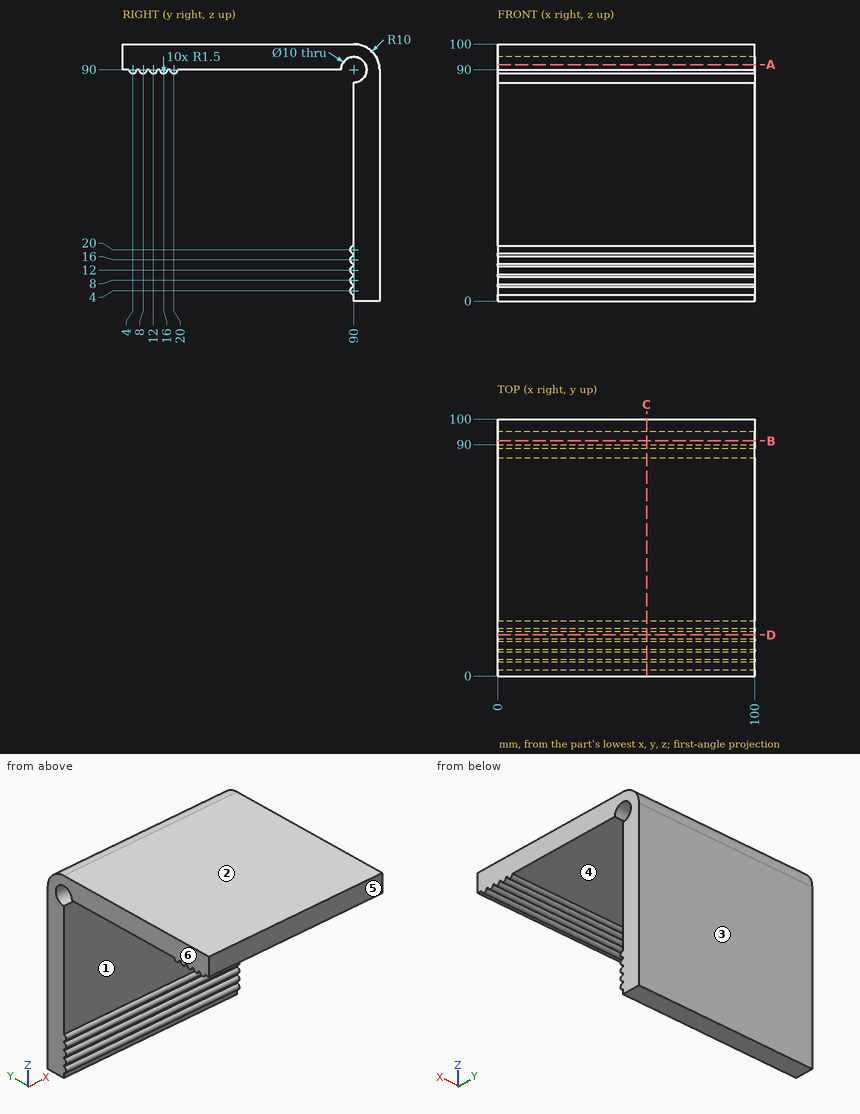
Source: three-view drawing plus pictorial views. Frame: mm from the lowest corner of the part. A direction names the side the tool comes from. Coordinates: 2 decimals unless noted, no trailing zeros. Loops run counter-clockwise (first coordinate to the right, second up) from the corner with the lowest first, then second, coordinate; pieces in that order, holes last. Notation, with made-up numbers: (72, 44) -> (120, 44) arc R4 ccw to (120, 50) -> close; hole circle Ø1 at (51.25, 86). An arc over 180 degrees is marked (long way). Answer in a Markdown table with one row per item. Add a question column.
Q1. Section A-A on z = 92. Return the cut outline in (x, y).
Q2. Reachability of the marked faces 1 and 2 from +Z, -Z, +X, -X, +Y, -Y: full face, straight path, thin tool, end or side. Return the list, or none.
Q3. Ray query, line 1 along Y through (x, z) = (60.5, 89); line 2 along Z through (x, y) = (83, 81). Return the intervals inside material, ascending.
Q4. Contact query for flat-ended pins moving along their axis: pin 1 Ø5 at (x, y) = (52, 43) entering from -Z; pin 2 Ø0.8 at (x, z) = (29, 6) entering from -Y. Output: stop coordinate, or through.
Q5. Section B-B on y = 91.5. Return the cut outline in (x, z).
Q6. Pull-direction query (Y, two-part tool) for the marked faces 3, 4, 5 and 6; classes: pulls with the +Y half, pulls with the -Y half, needs draft (parallel to the pull), parting line crosses it, or undercut.
Q7. Section C-C on x = 58. Return the cut outline in (y, z).
Q8. Section D-D on y = 16. Return the cut outline in (x, z), and give its area (3 significant figures).
Computed values:
| question | item | result |
|---|---|---|
| 1 | outline | (0, 0) -> (100, 0) -> (100, 85.42) -> (0, 85.42) -> close; (0, 94.58) -> (100, 94.58) -> (100, 99.8) -> (0, 99.8) -> close |
| 2 | face 1 | +X, -X, -Y |
| 2 | face 2 | +Z, +X, -X, +Y, -Y |
| 3 | line 1 | y = 2.88 to 5.12, 6.88 to 9.12, 10.88 to 13.12, 14.88 to 17.12, 18.88 to 21.12, 94.9 to 100 |
| 3 | line 2 | z = 90 to 100 |
| 4 | pin 1 | stops at z = 90 |
| 4 | pin 2 | stops at y = 90 |
| 5 | outline | (0, 0) -> (100, 0) -> (100, 85.23) -> (0, 85.23) -> close; (0, 94.77) -> (100, 94.77) -> (100, 99.89) -> (0, 99.89) -> close |
| 6 | face 3 | pulls with the +Y half |
| 6 | face 4 | undercut |
| 6 | face 5 | pulls with the -Y half |
| 6 | face 6 | needs draft |
| 7 | outline | (0, 90) -> (2.5, 90) arc R1.5 ccw to (5.5, 90) -> (6.5, 90) arc R1.5 ccw to (9.5, 90) -> (10.5, 90) arc R1.5 ccw to (13.5, 90) -> (14.5, 90) arc R1.5 ccw to (17.5, 90) -> (18.5, 90) arc R1.5 ccw to (21.5, 90) -> (85, 90) arc R5 cw (long way) to (90, 85) -> (90, 21.5) arc R1.5 ccw to (90, 18.5) -> (90, 17.5) arc R1.5 ccw to (90, 14.5) -> (90, 13.5) arc R1.5 ccw to (90, 10.5) -> (90, 9.5) arc R1.5 ccw to (90, 6.5) -> (90, 5.5) arc R1.5 ccw to (90, 2.5) -> (90, 0) -> (100, 0) -> (100, 90) arc R10 ccw to (90, 100) -> (0, 100) -> close |
| 8 | outline | (0, 88.5) -> (100, 88.5) -> (100, 100) -> (0, 100) -> close |
| 8 | area | 1,150 mm^2 |
